```python
from build123d import *

# Parameters (mm, degrees)
PAD_DEPTH    = 50
SKETCH003_W  = 20
SKETCH003_H  = 2.5
PAD001_DEPTH = 25
CHAMFER_SIZE = 19
SKETCH004_R  = 1.6
SKETCH004_W  = 19
SKETCH004_H  = 27.5
POCKET_DEPTH = 23.001
FILLET_R     = 3
SKETCH005_R  = 2.2
HOLE_DEPTH   = 25


with BuildPart() as part:
    # Sketch → Pad (new body)
    with BuildSketch(Plane.XZ):
        Polygon((-23, 3), (-23, 0), (0, 0), (0, 28), (-3, 28), (-3, 3), align=None)
    extrude(amount=PAD_DEPTH)

    # Sketch003 (on Face6 of Pad) → Pad001 (join)
    with BuildSketch(Plane(origin=(0, 0, 3), x_dir=(-1, 0, 0), z_dir=(0, 0, 1))):
        with Locations((13, 40.25)):
            Rectangle(SKETCH003_W, SKETCH003_H)
        with Locations((13, 9.75)):
            Rectangle(SKETCH003_W, SKETCH003_H)
    extrude(amount=PAD001_DEPTH)

    # Chamfer
    chamfer_edges = [part.edges().sort_by_distance(p)[0] for p in [
        (-23, -40.25, 28),
        (-23, -9.75, 28),
    ]]
    chamfer(chamfer_edges, length=CHAMFER_SIZE)

    # Sketch004 (on Face21 of Chamfer) → Pocket (cut, through all)
    with BuildSketch(Plane(origin=(0, 0, 0), x_dir=(0, 0, 1), z_dir=(1, 0, 0))):
        with Locations((14, 44.75)):
            Circle(SKETCH004_R)
        with Locations((14, 5.25)):
            Circle(SKETCH004_R)
        with Locations((14, 25)):
            Rectangle(SKETCH004_W, SKETCH004_H)
    extrude(amount=-POCKET_DEPTH, mode=Mode.SUBTRACT)

    # Fillet
    fillet_edges = [part.edges().sort_by_distance(p)[0] for p in [
        (-1.5, -11.25, 4.5),
        (-1.5, -11.25, 23.5),
        (-1.5, -38.75, 4.5),
        (-1.5, -38.75, 23.5),
    ]]
    fillet(fillet_edges, radius=FILLET_R)

    # Sketch005 (on Face9 of Pocket) → Hole (cut)
    with BuildSketch(Plane(origin=(0, 0, 3), x_dir=(-1, 0, 0), z_dir=(0, 0, 1))):
        with Locations((13, 4.25)):
            Circle(SKETCH005_R)
        with Locations((13, 45.75)):
            Circle(SKETCH005_R)
    extrude(amount=-HOLE_DEPTH, mode=Mode.SUBTRACT)


solid = part.part
```
Read the model definition and answer for the solid it produces. Units are mm, in the model's axes. A direction names the side the tool comes from. Give positions to 0.01 mm unless a question says otherwise; leave off trailing zeros. Write each loop counter-clockwise with the first axis right and the second up, starting at its lowest first coordinate (ties: lowest second). Pieces come first, ordered by that corner, then holes. Notation, with made-up numbers: (26.5, 5.5) - (34.5, 5.5) arc R28 ccw to (34.5, 37.5) - close; hole circle Ø7 at (-18.5, -2.75). An arc over 180 degrees is marked (long way). Write item = value, one per line. Start each with the question number.
Item 1: Find section B-B (x = -13). Give the vertices of the cut face in (y, z), then the cut area to 3 significant figures.
Item 2: Find section A-A (y = -27). Give the vertices of the cut face in (x, z), then the cut area to 3 significant figures.
Item 3: A tool of negligible diameter and unlimited length cuts with its end or side. For faces 4 (the flat face through (-3, -4, 16)), 5 (the flat face through (-1, -25, 23.5)), 6 (the flat face through (-11, -11, 13)), 7 (the flat face through (-3, -46, 16)), from which of +Z, -Z, +X, -X, +Y, -Y can it reach the whole face along a straight path? Write none if from no direction.
Item 4: Find the intervals of material crossed by probe 1 along Y at (x, z) = (-1.3, 14); probe 2 along Y at (x, z) = (-13, 2.1); probe 3 along X at (y, z) = (-45.75, 1.35), in increasing order. Write a range as [from, to].
Item 5: Find section D-D (z = 19). Give the vertices of the cut face in (x, y), then the cut area to 4 significant figures.
Item 6: Find section C-C (z = 14). Give the vertices of the cut face in (x, y).
Item 7: The mould has two halves that part along X. Classify faces 1 (the flat face through (-3, -25, 24)), 2 (the cylindrical face through (-12.523, -43.602, 1.521)), 3 (the cylindrical face through (-1.52, -12.11, 5.4)): +X half, -X half, draft (parallel to the pull), parting line (faces both ways), or undercut.
Item 8: Each of these flat-tipped pins is pushed along its axis until it touches: P1, Ø6, axis at x = -17.5, z = 13, coming from the +Y side; P2, Ø10, axis at y = -32.5, z = 20.5, coming from the -X side; P3, Ø6, axis at x = -9.5, z = 20, coming from the -Y side. Where does it stop, or does it pass through?
Response:
q1.outline = (-50, 0) - (-47.95, 0) - (-47.95, 3) - (-50, 3) - close; (-43.55, 0) - (-6.45, 0) - (-6.45, 3) - (-8.5, 3) - (-8.5, 19) - (-11, 19) - (-11, 3) - (-39, 3) - (-39, 19) - (-41.5, 19) - (-41.5, 3) - (-43.55, 3) - close; (-2.05, 0) - (0, 0) - (0, 3) - (-2.05, 3) - close
q1.area = 204 mm²
q2.outline = (-23, 0) - (0, 0) - (0, 4.5) - (-3, 4.5) - (-3, 3) - (-23, 3) - close; (-3, 23.5) - (0, 23.5) - (0, 28) - (-3, 28) - close
q2.area = 87.0 mm²
q3.face_4 = +Z, -X, +Y
q3.face_5 = +X, -X
q3.face_6 = +Z, -X
q3.face_7 = +Z, -X, -Y
q4.probe_1 = [-50, -46.35], [-43.15, -38.75], [-11.25, -6.85], [-3.65, 0]
q4.probe_2 = [-50, -47.95], [-43.55, -6.45], [-2.05, 0]
q4.probe_3 = [-23, -15.2], [-10.8, 0]
q5.outline = (-13, -41.5) - (-3, -41.5) - (-3, -50) - (0, -50) - (0, -38.75) - (-3, -38.75) - (-3, -39) - (-13, -39) - close; (-13, -11) - (-3, -11) - (-3, -11.25) - (0, -11.25) - (0, 0) - (-3, 0) - (-3, -8.5) - (-13, -8.5) - close
q5.area = 117.5 mm²
q6.outline = (-18, -41.5) - (-3, -41.5) - (-3, -43.15) - (0, -43.15) - (0, -38.75) - (-3, -38.75) - (-3, -39) - (-18, -39) - close; (-18, -11) - (-3, -11) - (-3, -11.25) - (0, -11.25) - (0, -6.85) - (-3, -6.85) - (-3, -8.5) - (-18, -8.5) - close; (-3, -50) - (0, -50) - (0, -46.35) - (-3, -46.35) - close; (-3, -3.65) - (0, -3.65) - (0, 0) - (-3, 0) - close
q7.face_1 = -X half
q7.face_2 = undercut
q7.face_3 = draft
q8.P1 = -8.5
q8.P2 = -3
q8.P3 = -41.5
